from build123d import *

# Parameters (mm, degrees)
SKETCH1_W           = 44
SKETCH1_H           = 8
SKETCH3_R           = 2
BOSS_EXTRUDE1_DEPTH = 12
SKETCH4_W           = 6
SKETCH4_H           = 8
SKETCH5_W           = 1.35
SKETCH5_H           = 2


with BuildPart() as part:
    # Sketch1 → Revolve1 (revolve)
    with BuildSketch(Plane.XY):
        with Locations((-3, 4)):
            Rectangle(SKETCH1_W, SKETCH1_H)
    revolve(axis=Axis((19, 0, 0), (-1, 0, 0)))

    # Sketch2 → Cut-Revolve1 (revolve, cut)
    with BuildSketch(Plane.XY):
        Polygon((-25, 6.5), (-23.5, 8), (-25, 8), align=None)
    revolve(axis=Axis((39, 0, 0), (-1, 0, 0)), mode=Mode.SUBTRACT)

    # Sketch3 → Boss-Extrude1 (add)
    with BuildSketch(Plane(origin=(0, 0, 0), x_dir=(1, 0, 0), z_dir=(0, 1, 0))):
        with Locations((-20, 0)):
            Circle(SKETCH3_R)
    extrude(amount=-BOSS_EXTRUDE1_DEPTH)

    # Sketch4 → Revolve2 (revolve)
    with BuildSketch(Plane.XY):
        with Locations((22, 4)):
            Rectangle(SKETCH4_W, SKETCH4_H)
    revolve(axis=Axis((25, 0, 0), (-1, 0, 0)))

    # Sketch5 → Cut-Revolve2 (revolve, cut)
    with BuildSketch(Plane.XY):
        with Locations((19.675, 7)):
            Rectangle(SKETCH5_W, SKETCH5_H)
    revolve(axis=Axis((39, 0, 0), (-1, 0, 0)), mode=Mode.SUBTRACT)

    # Sketch6 → Cut-Revolve3 (revolve, cut)
    with BuildSketch(Plane.XY):
        Polygon((23.5, 8), (25, 6.5), (25, 8), align=None)
    revolve(axis=Axis((39, 0, 0), (-1, 0, 0)), mode=Mode.SUBTRACT)


solid = part.part
Build history of the part. All positions in model axes, mm. A direction names the side the tool comes from. Coordinates: 2 decimals unless noted, no trailing zeros. Order: outer loops, then holes, each group sorted by start corner. A loop starts at its lowest first (then second) coordinate and runs counter-clockwise, first axis right, second up. Notation, with made-up numbers: (26.5, 56.5) -> (42.5, 56.5) arc R17 ccw to (42.5, 69.5) -> close; hole circle Ø3 at (53, 86.5). An arc over 180 degrees is marked (long way). One line per item, written item: value.
(1) Slice it at C-C, the plane x = -0.5. List the corners of the cut face in (y, z).
Checked values:
outline: circle Ø16 at (0, 0)
(2) Mould opens along X. For faces 4 (the flat face through (19, 2, -6)), 5 (the flat face through (-25, 0, 0)), 6 (the flat face through (25, 0, 0)), 7 (the cylindrical face through (21.95, -1.73, 7.81)) say: pulls with the +X half, pulls with the -X half, needs draft (parallel to the pull), parting line crosses it, or undercut.
Checked values:
face 4: undercut
face 5: pulls with the -X half
face 6: pulls with the +X half
face 7: needs draft
(3) Probe line 1 (X direction, y = 5.5, z = 4); line 2 (X direction, y = -4, z = 5); line 3 (Y direction, x = 13.5, z = -6.5). List the from-to ranges inside material, lowest first. Write a range as [from, to].
Checked values:
line 1: [-24.7, 19], [20.35, 24.7]
line 2: [-25, 19], [20.35, 25]
line 3: [-4.66, 4.66]
(4) Slice it at A-A, the plane z = 0. List the corners of the cut face in (x, y), plus the area to 3 significant figures.
Checked values:
outline: (-25, -6.5) -> (-23.5, -8) -> (-22, -8) -> (-22, -12) -> (-18, -12) -> (-18, -8) -> (19, -8) -> (19, -6) -> (20.35, -6) -> (20.35, -8) -> (23.5, -8) -> (25, -6.5) -> (25, 6.5) -> (23.5, 8) -> (20.35, 8) -> (20.35, 6) -> (19, 6) -> (19, 8) -> (-23.5, 8) -> (-25, 6.5) -> close
area: 806 mm2
(5) Slice it at B-B, the plane x = -20. List the corners of the cut face in (y, z), plus the area to 3 significant figures.
Checked values:
outline: (-12, -2) -> (-7.75, -2) arc R8 ccw (long way) to (-7.75, 2) -> (-12, 2) -> close
area: 217 mm2
(6) Tool access for faces 1 (the flat face through (-20, -12, 0)), 2 (the cylindrical face through (-22, -10, 0)), 3 (the cylindrical face through (20, -6, 0)): list every direction of +Z, -Z, +X, -X, +Y, -Y with a clear straight run to the whole face (end or side of a thin tool).
Checked values:
face 1: +Z, -Z, +X, -X, -Y
face 2: -Y
face 3: none
(7) Drop flat-ended pins along their axis: pin 1 Ø8 at (x, y) = (-9, -5) entering from +Z; pin 2 Ø6 at (x, y) = (-0.5, -5.5) entering from +Z; pin 3 Ø6 at (x, y) = (5, 4.5) entering from -Z. Give the stop position or say it passes through.
Checked values:
pin 1: z = 7.94
pin 2: z = 7.6
pin 3: z = -7.86
